For this review, take the finished solid that the model builds, in its own axes (mm). A direction names the side the tool comes from. Round coordinates to 2 decimals unless told otherwise and drop trailing zeros. Order: outer loops, then holes, each group sorted by start corner. A loop starts at its lowest first (then second) coordinate and runs counter-clockwise, first axis right, second up. Notation, with made-up numbers: M 88,-5 L 108,-5 A18 ccw 108,25 Z; hole C 28,-16.5 d1. An arc over 180 degrees is marked long. Answer in a Markdown table with one row per item. Add a question column.
```python
from build123d import *

# Parameters (mm, degrees)
SKETCH1_W           = 10
SKETCH1_H           = 20
SKETCH1_H_2         = 10
SKETCH1_W_2         = 20
BOSS_EXTRUDE1_DEPTH = 10
SKETCH2_W           = 10
SKETCH2_H           = 10
BOSS_EXTRUDE2_DEPTH = 93.5
SKETCH3_W           = 10
SKETCH3_H           = 20
SKETCH3_H_2         = 10
SKETCH3_W_2         = 20
BOSS_EXTRUDE3_DEPTH = 5
SKETCH4_W           = 20
SKETCH4_H           = 10
SKETCH4_W_2         = 10
SKETCH4_H_2         = 20
CUT_EXTRUDE1_DEPTH  = 5
SKETCH5_R           = 1.6
CUT_EXTRUDE2_DEPTH  = 1.2
SKETCH6_R           = 1.5
CUT_EXTRUDE3_DEPTH  = 10
SKETCH7_R           = 1.6
CUT_EXTRUDE4_DEPTH  = 1.2
SKETCH8_R           = 1.5
CUT_EXTRUDE5_DEPTH  = 10.2
SKETCH9_R           = 1.5
CUT_EXTRUDE6_DEPTH  = 10.2
SKETCH10_R          = 1.5
CUT_EXTRUDE7_DEPTH  = 12.2
SKETCH11_R          = 1.5
CUT_EXTRUDE8_DEPTH  = 10
CUT_EXTRUDE9_START  = -12
SKETCH12_R          = 1.5
CUT_EXTRUDE9_DEPTH  = 12
SKETCH13_R          = 1.6
CUT_EXTRUDE10_DEPTH = 1.2
SKETCH14_W          = 10
SKETCH14_H          = 5
BOSS_EXTRUDE4_DEPTH = 5
SKETCH15_W          = 10
SKETCH15_H          = 5
BOSS_EXTRUDE5_DEPTH = 5
SKETCH16_R          = 1.6
CUT_EXTRUDE11_DEPTH = 1.2


with BuildPart() as part:
    # Sketch1 → Boss-Extrude1 (new body)
    with BuildSketch(Plane(origin=(0, 0, 0), x_dir=(1, 0, 0), z_dir=(0, 1, 0))):
        with Locations((5, 20)):
            Rectangle(SKETCH1_W, SKETCH1_H)
        with Locations((5, 5)):
            Rectangle(SKETCH1_W, SKETCH1_H_2)
        with Locations((20, 5)):
            Rectangle(SKETCH1_W_2, SKETCH1_H_2)
    extrude(amount=BOSS_EXTRUDE1_DEPTH)

    # Sketch2 → Boss-Extrude2 (add)
    with BuildSketch(Plane(origin=(0, 10, 0), x_dir=(1, 0, 0), z_dir=(0, 1, 0))):
        with Locations((5, 5)):
            Rectangle(SKETCH2_W, SKETCH2_H)
    extrude(amount=BOSS_EXTRUDE2_DEPTH)

    # Sketch3 → Boss-Extrude3 (add)
    with BuildSketch(Plane(origin=(0, 103.5, 0), x_dir=(1, 0, 0), z_dir=(0, 1, 0))):
        with Locations((5, 20)):
            Rectangle(SKETCH3_W, SKETCH3_H)
        with Locations((5, 5)):
            Rectangle(SKETCH3_W, SKETCH3_H_2)
        with Locations((20, 5)):
            Rectangle(SKETCH3_W_2, SKETCH3_H_2)
    extrude(amount=BOSS_EXTRUDE3_DEPTH)

    # Sketch4 → Cut-Extrude1 (cut)
    with BuildSketch(Plane(origin=(0, 10, 0), x_dir=(1, 0, 0), z_dir=(0, 1, 0))):
        with Locations((20, 5)):
            Rectangle(SKETCH4_W, SKETCH4_H)
        with Locations((5, 20)):
            Rectangle(SKETCH4_W_2, SKETCH4_H_2)
    extrude(amount=-CUT_EXTRUDE1_DEPTH, mode=Mode.SUBTRACT)

    # Sketch5 → Cut-Extrude2 (cut)
    with BuildSketch(Plane.XY):
        with Locations((5, 5)):
            Circle(SKETCH5_R)
        with Locations((27.5, 2.5)):
            Circle(SKETCH5_R)
        with Locations((5, 15)):
            Circle(SKETCH5_R)
        with Locations((12.5, 2.5)):
            Circle(SKETCH5_R)
        with Locations(Location((27.5, 106, 0), (0, 0, 180))):
            Circle(SKETCH5_R)
        with Locations(Location((12.5, 106, 0), (0, 0, 180))):
            Circle(SKETCH5_R)
        with Locations(Location((5, 103.5, 0), (0, 0, 180))):
            Circle(SKETCH5_R)
        with Locations(Location((5, 93.5, 0), (0, 0, 180))):
            Circle(SKETCH5_R)
    extrude(amount=-CUT_EXTRUDE2_DEPTH, mode=Mode.SUBTRACT)

    # Sketch6 → Cut-Extrude3 (cut)
    with BuildSketch(Plane.XY):
        with Locations((20, 106)):
            Circle(SKETCH6_R)
        with Locations((5, 98.5)):
            Circle(SKETCH6_R)
        with Locations((5, 10)):
            Circle(SKETCH6_R)
        with Locations((20, 2.5)):
            Circle(SKETCH6_R)
    extrude(amount=-CUT_EXTRUDE3_DEPTH, mode=Mode.SUBTRACT)

    # Sketch7 → Cut-Extrude4 (cut)
    with BuildSketch(Plane.ZY):
        with Locations((-27.5, 106)):
            Circle(SKETCH7_R)
        with Locations((-12.5, 106)):
            Circle(SKETCH7_R)
        with Locations((-5, 103.5)):
            Circle(SKETCH7_R)
        with Locations((-5, 93.5)):
            Circle(SKETCH7_R)
        with Locations((-27.5, 2.5)):
            Circle(SKETCH7_R)
        with Locations((-12.5, 2.5)):
            Circle(SKETCH7_R)
        with Locations((-5, 5)):
            Circle(SKETCH7_R)
        with Locations((-5, 15)):
            Circle(SKETCH7_R)
    extrude(amount=-CUT_EXTRUDE4_DEPTH, mode=Mode.SUBTRACT)

    # Sketch8 → Cut-Extrude5 (cut)
    with BuildSketch(Plane.ZY):
        with Locations((-20, 106)):
            Circle(SKETCH8_R)
        with Locations((-5, 98.5)):
            Circle(SKETCH8_R)
        with Locations(Location((-5, 10, 0), (0, 0, 270))):
            Circle(SKETCH8_R)
        with Locations((-20, 2.5)):
            Circle(SKETCH8_R)
    extrude(amount=-CUT_EXTRUDE5_DEPTH, mode=Mode.SUBTRACT)

    # Sketch9 → Cut-Extrude6 (cut)
    with BuildSketch(Plane(origin=(0, 5, 0), x_dir=(1, 0, 0), z_dir=(0, 1, 0))):
        with Locations(Location((25, 5, 0), (0, 0, 270))):
            Circle(SKETCH9_R)
        with Locations(Location((15, 5, 0), (0, 0, 270))):
            Circle(SKETCH9_R)
        with Locations(Location((5, 15, 0), (0, 0, 270))):
            Circle(SKETCH9_R)
        with Locations(Location((5, 25, 0), (0, 0, 270))):
            Circle(SKETCH9_R)
    extrude(amount=-CUT_EXTRUDE6_DEPTH, mode=Mode.SUBTRACT)

    # Sketch10 → Cut-Extrude7 (cut)
    with BuildSketch(Plane.XZ):
        with Locations(Location((5, -5, 0), (0, 0, 270))):
            Circle(SKETCH10_R)
    extrude(amount=-CUT_EXTRUDE7_DEPTH, mode=Mode.SUBTRACT)

    # Sketch11 → Cut-Extrude8 (cut)
    with BuildSketch(Plane(origin=(0, 108.5, 0), x_dir=(1, 0, 0), z_dir=(0, 1, 0))):
        with Locations(Location((5, 15, 0), (0, 0, 270))):
            Circle(SKETCH11_R)
        with Locations(Location((5, 25, 0), (0, 0, 270))):
            Circle(SKETCH11_R)
        with Locations(Location((15, 5, 0), (0, 0, 270))):
            Circle(SKETCH11_R)
        with Locations(Location((25, 5, 0), (0, 0, 270))):
            Circle(SKETCH11_R)
    extrude(amount=-CUT_EXTRUDE8_DEPTH, mode=Mode.SUBTRACT)

    # Sketch12 → Cut-Extrude9 (cut)
    with BuildSketch(Plane(origin=(0, 108.5, 0), x_dir=(1, 0, 0), z_dir=(0, 1, 0)).offset(CUT_EXTRUDE9_START)):
        with Locations(Location((5, 5, 0), (0, 0, 90))):
            Circle(SKETCH12_R)
    extrude(amount=CUT_EXTRUDE9_DEPTH, mode=Mode.SUBTRACT)

    # Sketch13 → Cut-Extrude10 (cut)
    with BuildSketch(Plane(origin=(0, 108.5, 0), x_dir=(1, 0, 0), z_dir=(0, 1, 0))):
        with Locations(Location((10, 5, 0), (0, 0, 270))):
            Circle(SKETCH13_R)
        with Locations(Location((5, 10, 0), (0, 0, 270))):
            Circle(SKETCH13_R)
    extrude(amount=-CUT_EXTRUDE10_DEPTH, mode=Mode.SUBTRACT)

    # Sketch14 → Boss-Extrude4 (add)
    with BuildSketch(Plane(origin=(0, 0, -30), x_dir=(-1, 0, 0), z_dir=(0, 0, -1))):
        with Locations((-5, 106)):
            Rectangle(SKETCH14_W, SKETCH14_H)
    extrude(amount=BOSS_EXTRUDE4_DEPTH)

    # Sketch15 → Boss-Extrude5 (add)
    with BuildSketch(Plane(origin=(30, 0, 0), x_dir=(0, 0, -1), z_dir=(1, 0, 0))):
        with Locations((5, 106)):
            Rectangle(SKETCH15_W, SKETCH15_H)
    extrude(amount=BOSS_EXTRUDE5_DEPTH)

    # Sketch16 → Cut-Extrude11 (cut)
    with BuildSketch(Plane(origin=(0, 108.5, 0), x_dir=(1, 0, 0), z_dir=(0, 1, 0))):
        with Locations(Location((31, 5, 0), (0, 0, 270))):
            Circle(SKETCH16_R)
        with Locations(Location((5, 31, 0), (0, 0, 270))):
            Circle(SKETCH16_R)
    extrude(amount=-CUT_EXTRUDE11_DEPTH, mode=Mode.SUBTRACT)


solid = part.part
```
1. To check wall thickness, follow probe 1 along Y at (x, z) = (5, -2.35); probe 2 along Y at (x, z) = (27, -3); probe 3 along Y at (x, z) = (0.9, -12.5). State the ranges of each line that lie inside material, in increasing order. Write a range as [from, to].
2. Consider section B-B on x = 27.5. Write out the cut boundary in (y, z).
3. For faces 1 (the flat face through (5, 103.5, -22)), 2 (the flat face through (20, 5, -5)), 3 (the flat face through (5, 96.5, -5)), 4 (the flat face through (10, 106, -22)), list the 3-axis set-ups (+Z, -Z, +X, -X, +Y, -Y) from which the entire face can be reached by the end or side of a thin tool; tool diameter is ignored.
4. Clearance check with flat-ended pins moving along their axes: pin 1 Ø5 at (y, z) = (15, -5) entering from +X; pin 2 Ø1.6 at (y, z) = (106.5, -12) entering from -X; pin 3 Ø5.5 at (x, y) = (16.5, 105.5) entering from -Z. State where each tip first meets the part, or that it passes through.
5. The part is to be moulded in two halves that separate along Z. For faces 5 (the flat face through (1.2, 3, -28)), 6 (the flat face through (9, 108.5, -13)), 7 (the flat face through (5, 93, -1.2)), say which applies: pulls with the +Z half, pulls with the -Z half, needs draft (parallel to the pull), parting line crosses it, or undercut.
6. Consider section C-C on x = 20. Write out the cut boundary in (y, z).
7. Consider section D-D on y = 93.5. Write out the cut boundary in (x, z).
8. Consider section A-A on z = -20. Write out the cut boundary in (x, y), plus the area to 3 significant figures.
Solved:
| question | item | result |
|---|---|---|
| 1 | probe 1 | y = [0, 8.5], [11.5, 97], [100, 108.5] |
| 1 | probe 2 | y = [0, 5], [103.5, 108.5] |
| 1 | probe 3 | y = [0, 0.9], [4.1, 5], [103.5, 104.4], [107.6, 108.5] |
| 2 | outline | M 0,-10 L 5,-10 L 5,0 L 4.1,0 L 4.1,-1.2 L 0.9,-1.2 L 0.9,0 L 0,0 Z; M 103.5,-10 L 108.5,-10 L 108.5,0 L 107.6,0 L 107.6,-1.2 L 104.4,-1.2 L 104.4,0 L 103.5,0 Z |
| 3 | face 1 | -Z, +X, -X |
| 3 | face 2 | +Z, -Z, +X |
| 3 | face 3 | +Y |
| 3 | face 4 | -Z, +X, +Y, -Y |
| 4 | pin 1 | stops at x = 10 |
| 4 | pin 2 | stops at x = 1.2 |
| 4 | pin 3 | stops at z = -10 |
| 5 | face 5 | undercut |
| 5 | face 6 | needs draft |
| 5 | face 7 | pulls with the +Z half |
| 6 | outline | M 0,-10 L 1,-10 L 1,0 L 0,0 Z; M 4,-10 L 5,-10 L 5,0 L 4,0 Z; M 103.5,-10 L 104.5,-10 L 104.5,0 L 103.5,0 Z; M 107.5,-10 L 108.5,-10 L 108.5,0 L 107.5,0 Z |
| 7 | outline | M 0,-10 L 10,-10 L 10,0 L 6.6,0 L 6.6,-1.2 L 3.4,-1.2 L 3.4,0 L 0,0 L 0,-3.4 L 1.2,-3.4 L 1.2,-6.6 L 0,-6.6 Z |
| 8 | outline | M 0,0 L 10,0 L 10,1 L 0,1 Z; M 0,4 L 10,4 L 10,5 L 0,5 Z; M 0,103.5 L 10,103.5 L 10,104.5 L 0,104.5 Z; M 0,107.5 L 10,107.5 L 10,108.5 L 0,108.5 Z |
| 8 | area | 40.0 mm^2 |
